Model file for the job. Use its own axes, mm. A direction names the side the tool comes from. Coordinates: 2 decimals unless noted, no trailing zeros. Loops run counter-clockwise (first coordinate to the right, second up) from the corner with the lowest first, then second, coordinate; pieces in that order, holes last. Notation, with made-up numbers: (75.5, 72) -> (80.5, 72) arc R30 cw to (80.5, 110) -> close; hole circle Ø3 at (37, -27). An arc over 180 degrees is marked (long way). Use one line per item in the form item = value.
```python
from build123d import *

# Parameters (mm, degrees)
SKETCH2_R                = 5.5
BOSS_EXTRUDE1_DEPTH      = 29
SKETCH3_R                = 12
CUT_EXTRUDE2_DEPTH       = 14
SKETCH5_R                = 4
SKETCH5_R_2              = 2
BOSS_EXTRUDE2_DEPTH      = 1
BOSS_EXTRUDE2_DEPTH_BACK = 1
SKETCH6_R                = 12
CUT_EXTRUDE3_DEPTH       = 1


with BuildPart() as part:
    # Sketch2 → Boss-Extrude1 (new body)
    with BuildSketch(Plane(origin=(0, 0, 0), x_dir=(1, 0, 0), z_dir=(0, 1, 0))):
        with BuildLine():
            ThreePointArc((50.009794046, 41.311227393), (41.887297641, 57.884223181), (28.818508763, 70.916716976))
            ThreePointArc((28.818508763, 70.916716976), (13.814285335, 58.864855467), (32.908133208, 61.2729792))
            ThreePointArc((32.908133208, 61.2729792), (40.45496434, 51.34849017), (45.618872448, 40.00017771))
            Line((45.618872448, 40.00017771), (51.710808427, 16.848599978))
            Line((51.710808427, 16.848599978), (58.045348615, 14.398829975))
            Line((58.045348615, 14.398829975), (50.009794046, 41.311227393))
        make_face()
        with Locations((23.020672213, 62.769012309)):
            Circle(SKETCH2_R, mode=Mode.SUBTRACT)
    extrude(amount=BOSS_EXTRUDE1_DEPTH)

    # Sketch3 → Cut-Extrude2 (cut)
    with BuildSketch(Plane(origin=(0, 7, 0), x_dir=(-1, 0, 0), z_dir=(0, -1, 0))):
        Polygon((-39.772770103, 64.267022184), (-15.893793884, 42.042250192), (-0.061179653, 60.713204229), (-23.940155872, 82.937976221), align=None)
        with Locations((-23.020672213, 62.769012309)):
            Circle(SKETCH3_R, mode=Mode.SUBTRACT)
        with BuildLine():
            ThreePointArc((-11.020672213, 62.769012309), (-24.725973403, 74.647225468), (-34.535996855, 59.393023803))
            Line((-34.535996855, 59.393023803), (-25.562701432, 51.041348968))
            ThreePointArc((-25.562701432, 51.041348968), (-15.487557008, 53.428125022), (-11.020672213, 62.769012309))
        make_face()
        with BuildLine():
            Line((-25.562701432, 51.041348968), (-34.535996855, 59.393023803))
            ThreePointArc((-34.535996855, 59.393023803), (-31.196240544, 53.984931113), (-25.562701432, 51.041348968))
        make_face()
    extrude(amount=-CUT_EXTRUDE2_DEPTH, mode=Mode.SUBTRACT)

    # Sketch5 → Boss-Extrude2 (add, two sides)
    with BuildSketch(Plane(origin=(0, 14.5, 0), x_dir=(-1, 0, 0), z_dir=(0, -1, 0))) as boss_extrude2_sk:
        with Locations((-48.811207054, 27.868142339)):
            Circle(SKETCH5_R)
        with Locations((-48.811207054, 27.868142339)):
            Circle(SKETCH5_R_2, mode=Mode.SUBTRACT)
    extrude(amount=BOSS_EXTRUDE2_DEPTH)
    extrude(boss_extrude2_sk.sketch, amount=-BOSS_EXTRUDE2_DEPTH_BACK)

    # Sketch6 → Cut-Extrude3 (cut)
    with BuildSketch(Plane(origin=(0, 22, 0), x_dir=(1, 0, 0), z_dir=(0, 1, 0))):
        Polygon((39.538971905, 63.831822433), (17.017916797, 43.859723681), (2.667298857, 64.33781743), (24.409587021, 83.619290887), align=None)
        with Locations((23.020672213, 62.769012309)):
            Circle(SKETCH6_R, mode=Mode.SUBTRACT)
        with BuildLine():
            ThreePointArc((24.993041452, 50.932215463), (30.982651495, 53.790878543), (34.536814652, 59.395814522))
            Line((34.536814652, 59.395814522), (24.993041452, 50.932215463))
        make_face()
        with BuildLine():
            Line((24.993041452, 50.932215463), (34.536814652, 59.395814522))
            ThreePointArc((34.536814652, 59.395814522), (34.899091916, 61.065150413), (35.020672213, 62.769012309))
            ThreePointArc((35.020672213, 62.769012309), (13.86456958, 70.525672967), (24.993041452, 50.932215463))
        make_face()
    extrude(amount=-CUT_EXTRUDE3_DEPTH, mode=Mode.SUBTRACT)


solid = part.part
```
Q1. Band-saw the part on C-C, the plane z = -28.5. Write the cut outline in (x, y) (3 decimals).
Result:
outline = (44.861, 13.5) -> (46.914, 13.5) -> (46.914, 15.5) -> (44.861, 15.5) -> close; (48.645, 0) -> (53.835, 0) -> (53.835, 29) -> (48.645, 29) -> close
Q2. Which spindle directions (+Z, -Z, +X, -X, +Y, -Y) get a long thin tool onto all of the face, cutting with end or side? Do faces 1 (the face through (36.38, 21.51, -61.03)), 2 (the face through (39, 0, -55)), 3 (the face through (46.8, 13.5, -27)). Say none if no direction does.
Result:
face_1 = -Z, -X
face_2 = +Z, -Z, +X, -X, -Y
face_3 = +Z, -X, -Y
Q3. Pin check, flat tips, straight feed: pin 1 Ø8 at (x, y) = (49.5, 22.5) entering from +Z; pin 2 Ø3 at (y, z) = (11.5, -56) entering from -X; pin 3 Ø4 at (y, z) = (22, -48.5) entering from -X. Stop position of each tip, or through.
Result:
pin_1 = -16.16
pin_2 = 36.2
pin_3 = 40.95
Q4. Band-saw the part on A-A, the plane z = -54.5. Write the cut outline in (x, y).
Result:
outline = (17.4, 0) -> (28.64, 0) -> (28.64, 7) -> (17.4, 7) -> close; (17.4, 22) -> (28.64, 22) -> (28.64, 29) -> (17.4, 29) -> close; (38.43, 0) -> (44.13, 0) -> (44.13, 29) -> (38.43, 29) -> close
Q5. Band-saw the part on B-B, the plane x = 21.5. Write the cut outline in (y, z), and give its area (3 significant figures).
Result:
outline = (0, -72.65) -> (7, -72.65) -> (7, -68.05) -> (0, -68.05) -> close; (0, -57.48) -> (7, -57.48) -> (7, -52.89) -> (0, -52.89) -> close; (22, -72.65) -> (29, -72.65) -> (29, -68.05) -> (22, -68.05) -> close; (22, -57.48) -> (29, -57.48) -> (29, -52.89) -> (22, -52.89) -> close
area = 129 mm2
Q6. Band-saw the part on D-D, the plane x = 29.5. Write the cut outline in (y, z).
Result:
outline = (0, -70.42) -> (7, -70.42) -> (7, -55.15) -> (0, -55.15) -> close; (22, -70.42) -> (29, -70.42) -> (29, -55.15) -> (22, -55.15) -> close
Q7. Mould opens along Y. For faces 4 (the face through (28.5, 7, -65.1)), 5 (the face through (18.97, 25.45, -66.49)), 6 (the face through (46.8, 15.5, -27)) say: released by +Y, released by -Y, zero draft, split by the parting line, or undercut.
Result:
face_4 = undercut
face_5 = zero draft
face_6 = released by +Y
Q8. Wall check: line 1 along X through (y, z) = (23, -61.5); line 2 along X through (y, z) = (26, -54.5); line 3 along Y through (x, z) = (45.5, -28). Give the ranges that are in metal, low to high.
Result:
line_1 = 13.1 to 17.67, 28.37 to 39.07
line_2 = 17.4 to 28.64, 38.43 to 44.13
line_3 = 13.5 to 15.5
